Design review of the part built by this model. Coordinates are the model's own, in mm. Face numbers are marked on the shaded views. A direction names the side the tool comes from. Give positions to 0.01 mm unless a question says otherwise; leave off trailing zeros. Order: outer loops, then holes, each group sorted by start corner. A loop starts at its lowest first (then second) coordinate and runs counter-clockwise, first axis right, second up. Notation, with made-up numbers: M 47,-34 L 75,-34 A10 ccw 75,-20 Z; hole C 5,60 d1. An arc over 180 degrees is marked long. Answer as a JSON object with one key per item and string values.
from build123d import *

# Parameters (mm, degrees)
BOSS_EXTRUDE1_DEPTH     = 40
BOSS_EXTRUDE2_START     = 30
SKETCH2_R               = 1.25
BOSS_EXTRUDE2_DEPTH     = 10
CUT_EXTRUDE1_START      = -30
SKETCH3_W               = 5
SKETCH3_H               = 5
CUT_EXTRUDE1_DEPTH      = 10
CUT_EXTRUDE2_DEPTH      = 110.544511501
CUT_EXTRUDE2_DEPTH_BACK = 110.544511501
SKETCH4_R               = 1.25
FILLET1_R               = 2.5


with BuildPart() as part:
    # Sketch1 → Boss-Extrude1 (new, symmetric)
    with BuildSketch(Plane.XY):
        Polygon((0, 0), (100, 0), (100, 20), (95, 20), (95, 5), (0, 5), align=None)
    extrude(amount=BOSS_EXTRUDE1_DEPTH, both=True)

    # Sketch2 → Boss-Extrude2 (add)
    with BuildSketch(Plane.XY.offset(BOSS_EXTRUDE2_START)):
        with BuildLine():
            Line((0, 5), (-2.5, 5))
            ThreePointArc((-2.5, 5), (-5, 2.5), (-2.5, 0))
            Line((-2.5, 0), (0, 0))
            Line((0, 0), (0, 5))
        make_face()
        with Locations((-2.5, 2.5)):
            Circle(SKETCH2_R, mode=Mode.SUBTRACT)
    boss_extrude2 = extrude(amount=BOSS_EXTRUDE2_DEPTH)

    # Mirror2: Boss-Extrude2 across plane
    add(boss_extrude2.mirror(Plane.XY))

    # Sketch3 → Cut-Extrude1 (cut)
    with BuildSketch(Plane.XY.offset(CUT_EXTRUDE1_START)):
        with Locations((97.5, 17.5)):
            Rectangle(SKETCH3_W, SKETCH3_H)
    cut_extrude1 = extrude(amount=-CUT_EXTRUDE1_DEPTH, mode=Mode.SUBTRACT)

    # Mirror3: Cut-Extrude1 across plane
    add(cut_extrude1.mirror(Plane.XY), mode=Mode.SUBTRACT)

    # Sketch4 → Cut-Extrude2 (cut, two sides: drawn at the far end of the back side and taken through both)
    with BuildSketch(Plane.XY.offset(-CUT_EXTRUDE2_DEPTH_BACK)):
        with Locations((97.5, 17.5)):
            Circle(SKETCH4_R)
    extrude(amount=CUT_EXTRUDE2_DEPTH + CUT_EXTRUDE2_DEPTH_BACK, mode=Mode.SUBTRACT)

    # Fillet1
    fillet1_edges = [part.edges().sort_by_distance(p)[0] for p in [
        (95, 20, 0),
        (100, 20, 0),
    ]]
    fillet(fillet1_edges, radius=FILLET1_R - 0.0001)  # a hair under: the kernel refuses the full size


solid = part.part
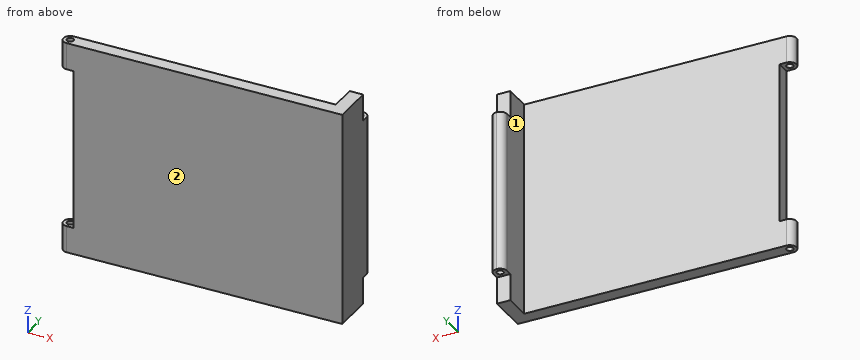
(1) To check wall thickness, follow L1, parallel to X at y = 17.5, z = -17; L2, parallel to Y at x = -2.5, z = -36.75; L3, parallel to Y at x = 80, z = -21. State the ranges of each line that lie inside material, in increasing order. Write a range as from..to.
Checked values:
{"L1": "x = 95..96.25, 98.75..100", "L2": "y = 0..1.25, 3.75..5", "L3": "y = 0..5"}
(2) We need section C-C (y = 7.25). Write out the cut boundary in (x, z), plus the area to 3 significant figures.
Checked values:
{"outline": "M 95,-40 L 100,-40 L 100,40 L 95,40 Z", "area": "400 mm^2"}
(3) Tool access review of the marked faces 1 and 2: name each direction out of +Z, -Z, +X, -X, +Y, -Y from which nothing blocks a thin tool from reaching the whole face with its end or side.
Checked values:
{"face 1": "+Z, -Z, -X, +Y", "face 2": "+Z, -Z, +X, -X, -Y"}
(4) Insertion check: pin 1 (6.5 mm diameter, centred on y = 13.5, z = -4.5, fed in from -X); pin 2 (6 mm diameter, centred on x = 77.5, z = -13, fed in from +Y); pin 3 (2.5 mm diameter, centred on y = 2.5, z = 6, fed in from -X). Each pin has a flat end and moves straight along its axis. Give the tip position at first contact, or say it passes through.
Checked values:
{"pin 1": "stops at x = 95", "pin 2": "stops at y = 5", "pin 3": "stops at x = 0"}
(5) We need section B-B (x = 20.5). Write out the cut boundary in (y, z), plus the area to 3 significant figures.
Checked values:
{"outline": "M 0,-40 L 5,-40 L 5,40 L 0,40 Z", "area": "400 mm^2"}
